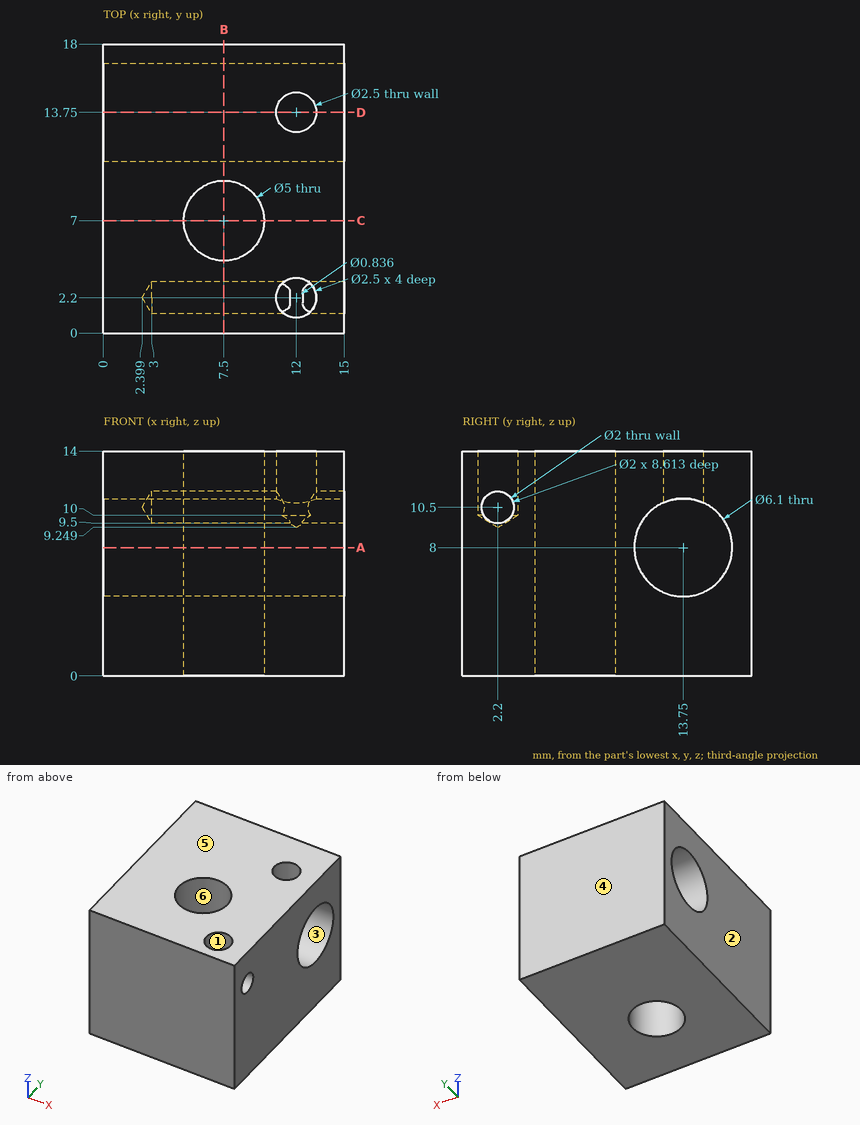
Input: dimensioned drawing with shaded views. Units: mm. Origin: part minimum x, y, z. A direction names the side the tool comes from. Round coordinates to 2 decimals unless told otherwise and drop trailing zeros. Loops run counter-clockwise (first coordinate to the right, second up) from the corner with the lowest first, then second, coordinate; pieces in that order, holes last. Notation, with made-up numbers: (54.25, 48) -> (97.25, 48) arc R16 ccw to (97.25, 56) -> close; hole circle Ø6 at (78.25, 47). An arc over 180 degrees is marked (long way). Use one line per item in the form item = value. Start each with the question number.
1) Section D-D on y = 13.75. Output: boundary loops of the cut face in (x, z).
2) Line query: L1, parallel to Y at x = 12, z = 12.9; L2, parallel to Z at x = 13.95, y = 2.2; L3, parallel to Y at x = 13.5, z = 10.5 (1 decimal). Output: solid intervals per line, ascending.
3) Draft query along Y for the marked faces 3, 4, 5 and 6. Return one class per face: released by +Y, released by -Y, zero draft, split by the parting line, or undercut.
4) Access query for the marked faces 1 and 2. Directions: +Z, -Z, +X, -X, +Y, -Y. A direction counts if a zero-diameter tool reaches every point of the face in a straight line with its end or side. Return the directions, or none.
5) First-contact query: P1, Ø2, axis at x = 12, y = 13.75, coming from the +Z side; P2, Ø5.5, axis at y = 13.75, z = 8, coming from the -X side; P3, Ø1.2, axis at y = 2.2, z = 10.5, coming from the +X side. Flat tips, straight axial feed; report the tip coordinate or a pass-through.
6) Section A-A on z = 8. Output: boundary loops of the cut face in (x, y), then the cut area to 3 significant figures.
7) Section B-B on x = 7.5. Output: boundary loops of the cut face in (y, z).
8) Section C-C on y = 7. Output: boundary loops of the cut face in (x, z), then the cut area to 3 significant figures.
Response:
q1.outline = (0, 0) -> (15, 0) -> (15, 4.95) -> (0, 4.95) -> close; (0, 11.05) -> (10.75, 11.05) -> (10.75, 14) -> (0, 14) -> close; (13.25, 11.05) -> (15, 11.05) -> (15, 14) -> (13.25, 14) -> close
q2.L1 = 0 to 0.95, 3.45 to 12.5, 15 to 18
q2.L2 = 0 to 9.5, 11.5 to 14
q2.L3 = 0 to 1.2, 3.2 to 12, 15.5 to 18
q3.face_3 = undercut
q3.face_4 = released by +Y
q3.face_5 = zero draft
q3.face_6 = undercut
q4.face_1 = +Z
q4.face_2 = +Z, -Z, -X, +Y, -Y
q5.P1 = 5.12
q5.P2 = through
q5.P3 = 2.76
q6.outline = (0, 0) -> (15, 0) -> (15, 10.7) -> (0, 10.7) -> close; (0, 16.8) -> (15, 16.8) -> (15, 18) -> (0, 18) -> close; hole circle Ø5 at (7.5, 7)
q6.area = 159 mm^2
q7.outline = (0, 0) -> (4.5, 0) -> (4.5, 14) -> (0, 14) -> close; (9.5, 0) -> (18, 0) -> (18, 14) -> (9.5, 14) -> close; hole circle Ø2 at (2.2, 10.5); hole circle Ø6.1 at (13.75, 8)
q8.outline = (0, 0) -> (5, 0) -> (5, 14) -> (0, 14) -> close; (10, 0) -> (15, 0) -> (15, 14) -> (10, 14) -> close
q8.area = 140 mm^2
